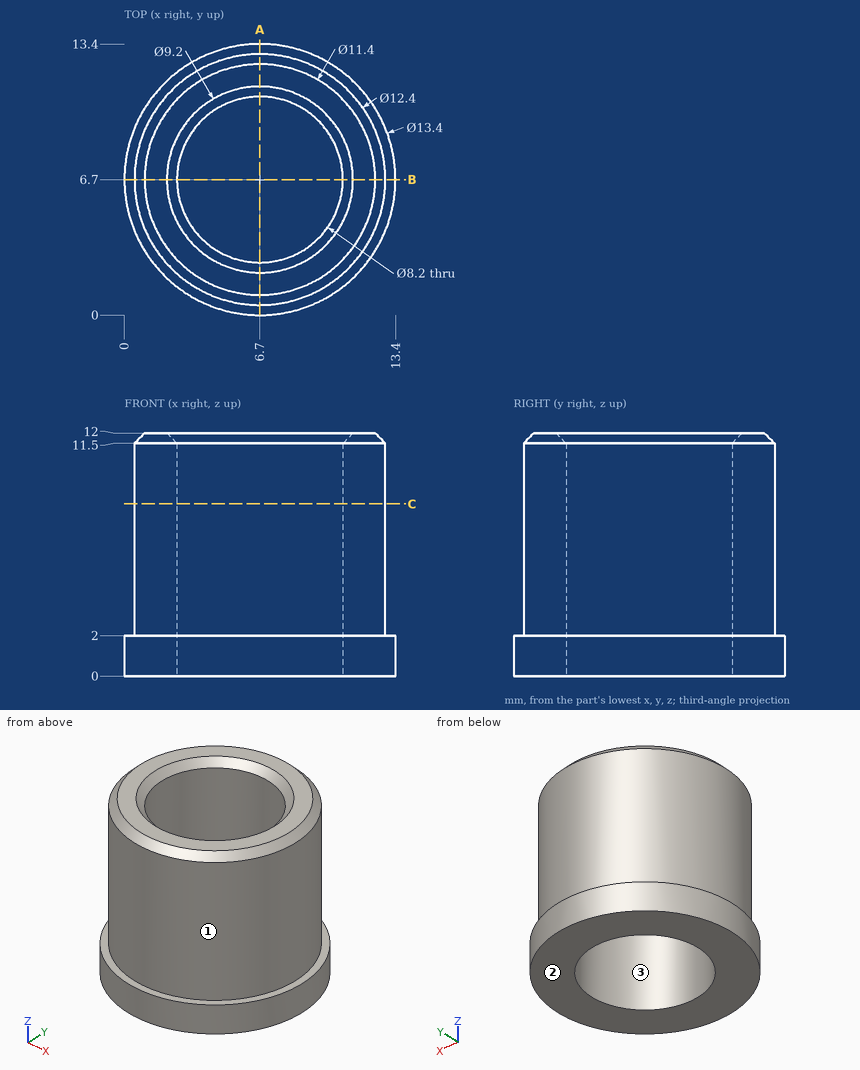
Design review of the part shown in the three views and the two pictorial views. Dimensions are in mm from the part's minimum x, y and z. Coordinates: 2 decimals unless noted, no trailing zeros. Loops run counter-clockwise (first coordinate to the right, second up) from the corner with the lowest first, then second, coordinate; pieces in that order, holes last.
(1) Insertion check: P1, Ø2, axis at y = 11.5, z = 4.5, coming from the -X side; P2, Ø2, axis at x = 12, z = 9, coming from the +Y side; P3, Ø2, axis at y = 4, z = 5.5, coming from the -X side. Each pin has a flat end and moves straight along its axis. Give the tip position at first contact, or say it passes through.
Determined:
P1: stops at x = 1.8
P2: stops at y = 11.17
P3: stops at x = 0.74
(2) Draft analysis for pull direction Y (two halves, no side actions). For the marked faces 1, 2 and 3, state which applies: +Y half, -Y half, draft (parallel to the pull), parting line (faces both ways), or undercut.
Determined:
face 1: parting line
face 2: draft
face 3: undercut
(3) Wall thickness on L1, parallel to Y at x = 6.7, z = 7.5; L2, parallel to X at y = 9.5, z = 3.5 (3 decimals): over which ranges is each line inside the solid? List them lowest first.
Determined:
L1: y = 0.5 to 2.6, 10.8 to 12.9
L2: x = 1.168 to 3.705, 9.695 to 12.232
(4) Consider section C-C, the plane z = 8.5. Give the boundary of the cut face in (x, y).
Determined:
outline: circle Ø12.4 at (6.7, 6.7); hole circle Ø8.2 at (6.7, 6.7)
(5) Consider section A-A, the plane x = 6.7. Give the boundary of the cut face in (y, z), plus the area to 3 significant figures.
Determined:
outline: (0, 0) - (2.6, 0) - (2.6, 11.5) - (2.1, 12) - (1, 12) - (0.5, 11.5) - (0.5, 2) - (0, 2) - close; (10.8, 0) - (13.4, 0) - (13.4, 2) - (12.9, 2) - (12.9, 11.5) - (12.4, 12) - (11.3, 12) - (10.8, 11.5) - close
area: 51.9 mm2
